Part model, mm, in its own coordinate system. Coordinates: 2 decimals unless noted, no trailing zeros. Order: outer loops, then holes, each group sorted by start corner. A loop starts at its lowest first (then second) coordinate and runs counter-clockwise, first axis right, second up.
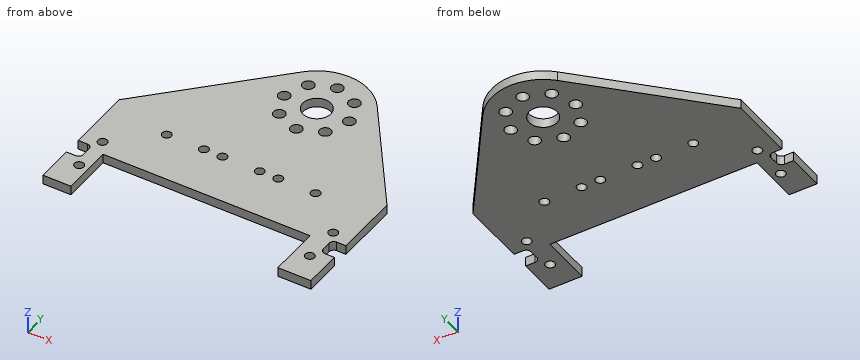
```python
from build123d import *

# Parameters (mm, degrees)
SKETCH_1_R      = 3
SKETCH_1_R_2    = 1.25
SKETCH_1_R_3    = 1
EXTRUDE_1_DEPTH = 2


with BuildPart() as part:
    # 草圖1 → 填料-伸長1 (new body)
    with BuildSketch(Plane.XY):
        with BuildLine():
            Line((25.8, -18), (25.8, -17))
            Line((25.8, -17), (8.925896882, 6.428714091))
            ThreePointArc((8.925896882, 6.428714091), (0.800566406, 10.970829204), (-7.898074186, 7.656397596))
            Line((-7.898074186, 7.656397596), (-31.8, -17))
            Line((-31.8, -17), (-31.8, -18))
            Line((-31.8, -18), (-31.8, -31))
            Line((-31.8, -31), (-29.8, -31))
            ThreePointArc((-29.8, -31), (-29.092893219, -31.292893219), (-28.8, -32))
            Line((-28.8, -32), (-28.8, -34))
            ThreePointArc((-28.8, -34), (-29.092893219, -34.707106781), (-29.8, -35))
            Line((-29.8, -35), (-31.8, -35))
            Line((-31.8, -35), (-31.8, -36))
            Line((-31.8, -36), (-31.8, -42))
            Line((-31.8, -42), (-31.8, -43))
            Line((-31.8, -43), (-30.8, -43))
            Line((-30.8, -43), (-26.8, -43))
            Line((-26.8, -43), (-25.8, -43))
            Line((-25.8, -43), (-25.8, -32))
            Line((-25.8, -32), (18.7, -32))
            Line((18.7, -32), (18.7, -43))
            Line((18.7, -43), (19.7, -43))
            Line((19.7, -43), (20.7, -43))
            Line((20.7, -43), (24.8, -43))
            Line((24.8, -43), (25.8, -43))
            Line((25.8, -43), (25.8, -42))
            Line((25.8, -42), (25.8, -36))
            Line((25.8, -36), (25.8, -35))
            Line((25.8, -35), (23.8, -35))
            ThreePointArc((23.8, -35), (23.092893219, -34.707106781), (22.8, -34))
            Line((22.8, -34), (22.8, -32))
            ThreePointArc((22.8, -32), (23.092893219, -31.292893219), (23.8, -31))
            Line((23.8, -31), (25.8, -31))
            Line((25.8, -31), (25.8, -18))
        make_face()
        Circle(SKETCH_1_R, mode=Mode.SUBTRACT)
        with Locations((0, 7)):
            Circle(SKETCH_1_R_2, mode=Mode.SUBTRACT)
        with Locations((4.949747468, 4.949747468)):
            Circle(SKETCH_1_R_2, mode=Mode.SUBTRACT)
        with Locations((7, 0)):
            Circle(SKETCH_1_R_2, mode=Mode.SUBTRACT)
        with Locations((4.949747468, -4.949747468)):
            Circle(SKETCH_1_R_2, mode=Mode.SUBTRACT)
        with Locations((0, -7)):
            Circle(SKETCH_1_R_2, mode=Mode.SUBTRACT)
        with Locations((-4.949747468, -4.949747468)):
            Circle(SKETCH_1_R_2, mode=Mode.SUBTRACT)
        with Locations((-7, 0)):
            Circle(SKETCH_1_R_2, mode=Mode.SUBTRACT)
        with Locations((-4.949747468, 4.949747468)):
            Circle(SKETCH_1_R_2, mode=Mode.SUBTRACT)
        with Locations((-27.8, -29)):
            Circle(SKETCH_1_R_3, mode=Mode.SUBTRACT)
        with Locations((-27.8, -37)):
            Circle(SKETCH_1_R_3, mode=Mode.SUBTRACT)
        with Locations(Location((21.8, -37, 0), (0, 0, 180))):
            Circle(SKETCH_1_R_3, mode=Mode.SUBTRACT)
        with Locations(Location((21.8, -29, 0), (0, 0, 180))):
            Circle(SKETCH_1_R_3, mode=Mode.SUBTRACT)
        with Locations((-19.05, -21)):
            Circle(SKETCH_1_R_3, mode=Mode.SUBTRACT)
        with Locations((-11.05, -21)):
            Circle(SKETCH_1_R_3, mode=Mode.SUBTRACT)
        with Locations((4.95, -21)):
            Circle(SKETCH_1_R_3, mode=Mode.SUBTRACT)
        with Locations((12.95, -21)):
            Circle(SKETCH_1_R_3, mode=Mode.SUBTRACT)
        with Locations((-7.05, -21)):
            Circle(SKETCH_1_R_3, mode=Mode.SUBTRACT)
        with Locations((0.95, -21)):
            Circle(SKETCH_1_R_3, mode=Mode.SUBTRACT)
    extrude(amount=EXTRUDE_1_DEPTH)


solid = part.part
```
(1) Probe line 1 (Y direction, x = -27.8, z = 1.3); line 2 (X direction, y = -5, z = 0.4); line 3 (Y direction, x = -4, z = 1.05). List the from-to ranges inside material, lowest first.
(2) Slice it at C-C, the plane x = 21.8. Give the cut face in (y, z).
(3) Slice it at A-A, the plane y = 0. Give the cut face in (x, z), then the cut area to 3 significant figures.
(4) Slice it at B-B, the plane x = -19.05. Give the cut face in (y, z).
(5) Drop flat-ended pins along their axis: pin 1 (1 mm diameter, centred on y = -33, z = 1.5, fed in from +X); pin 2 (1 mm diameter, centred on x = -7.5, z = 1.5, fed in from -Y). Give the stop position or say it passes through.
(6) Slice it at D-D, the plane x = -11.05. Give the cut face in (y, z).
Here are the results:
1. line 1: y = -43 to -38, -36 to -30, -28 to -12.87
1. line 2: x = -20.17 to -6.2, -3.7 to 3.7, 6.2 to 17.16
1. line 3: y = -32 to -5.76, -4.14 to 4.14, 5.76 to 10.25
2. outline: (-43, 0) - (-38, 0) - (-38, 2) - (-43, 2) - close; (-36, 0) - (-30, 0) - (-30, 2) - (-36, 2) - close; (-28, 0) - (-11.45, 0) - (-11.45, 2) - (-28, 2) - close
3. outline: (-15.32, 0) - (-8.25, 0) - (-8.25, 2) - (-15.32, 2) - close; (-5.75, 0) - (-3, 0) - (-3, 2) - (-5.75, 2) - close; (3, 0) - (5.75, 0) - (5.75, 2) - (3, 2) - close; (8.25, 0) - (13.56, 0) - (13.56, 2) - (8.25, 2) - close
3. area: 35.8 mm2
4. outline: (-32, 0) - (-22, 0) - (-22, 2) - (-32, 2) - close; (-20, 0) - (-3.85, 0) - (-3.85, 2) - (-20, 2) - close
5. pin 1: stops at x = 22.8
5. pin 2: stops at y = -32
6. outline: (-32, 0) - (-22, 0) - (-22, 2) - (-32, 2) - close; (-20, 0) - (4.4, 0) - (4.4, 2) - (-20, 2) - close
